Source: CAD feature listing. Evaluate the final solid. Frame: model axes, mm. Give positions to 0.01 mm unless a question says otherwise; leave off trailing zeros. Order: outer loops, then holes, each group sorted by start corner. A loop starts at its lowest first (then second) coordinate and runs counter-clockwise, first axis right, second up.
from build123d import *

# Parameters (mm, degrees)
SKETCH1_R           = 5.5
SKETCH1_R_2         = 4.7
BOSS_EXTRUDE1_DEPTH = 40
SKETCH2_R           = 5.5
BOSS_EXTRUDE2_DEPTH = 2
CHAMFER1_SIZE       = 1


with BuildPart() as part:
    # Sketch1 → Boss-Extrude1 (new body)
    with BuildSketch(Plane.XY):
        Circle(SKETCH1_R)
        Circle(SKETCH1_R_2, mode=Mode.SUBTRACT)
    extrude(amount=BOSS_EXTRUDE1_DEPTH)

    # Sketch2 → Boss-Extrude2 (add)
    with BuildSketch(Plane.XY.offset(40)):
        Circle(SKETCH2_R)
    extrude(amount=-BOSS_EXTRUDE2_DEPTH)

    # Chamfer1
    chamfer1_edges = [part.edges().sort_by_distance(p)[0] for p in [
        (-5.5, 0, 40),
    ]]
    chamfer(chamfer1_edges, length=CHAMFER1_SIZE)


solid = part.part
1) Section query C-C on z = 12. Output: boundary loops of the cut face in (x, y), and give its area (3 significant figures).
Checks:
outline: circle Ø11 at (0, 0); hole circle Ø9.4 at (0, 0)
area: 25.6 mm2
2) First-contact query: pin 1 Ø6 at (x, z) = (0.5, 27) entering from +Y; pin 2 Ø2 at (x, z) = (2, 14) entering from -Y; pin 3 Ø2 at (x, y) = (-3.5, 1) entering from -Z. Flat tips, straight axial feed; report the tip coordinate or a pass-through.
Checks:
pin 1: stops at y = 5.5
pin 2: stops at y = -5.41
pin 3: stops at z = 38
3) Pull-direction query (X, two-part tool) for faces 1 (the face through (0, 0, 40)), 2 (the face through (0, 0, 38)), 3 (the face through (-1.19, -5.37, 19.23)); classes: +X half, -X half, draft (parallel to the pull), parting line (faces both ways), or undercut.
Checks:
face 1: draft
face 2: undercut
face 3: parting line
4) Section query A-A on y = 0. Output: boundary loops of the cut face in (x, z).
Checks:
outline: (-5.5, 0) - (-4.7, 0) - (-4.7, 38) - (4.7, 38) - (4.7, 0) - (5.5, 0) - (5.5, 39) - (4.5, 40) - (-4.5, 40) - (-5.5, 39) - close
5) Ray query, L1, parallel to Y at x = 0, z = 12; L2, parallel to Z at x = -3.75, y = -0.75; L3, parallel to X at y = 2.75, z = 5. Return the intervals inside material, ascending.
Checks:
L1: y = -5.5 to -4.7, 4.7 to 5.5
L2: z = 38 to 40
L3: x = -4.76 to -3.81, 3.81 to 4.76
